```python
from build123d import *

# Parameters (mm, degrees)
F1_DEPTH = 20
F2_F1_R  = 2
F2_F2_R  = 2
F2_F3_R  = 2


with BuildPart() as f1:
    # F0 (on Top) → F1 (new body)
    with BuildSketch(Plane.XY):
        with BuildLine():
            ThreePointArc((0, 3.4753886408), (-6.702786735, 6.3139324677), (-9.1361551027, -0.5463444553))
            Line((-9.1361551027, -0.5463444553), (0, -18.3376532868))
            Line((0, -18.3376532868), (9.1361551027, -0.5463444553))
            ThreePointArc((9.1361551027, -0.5463444553), (6.702786735, 6.3139324677), (0, 3.4753886408))
        make_face()
        with BuildLine():
            ThreePointArc((0, 0), (-0.3116721052, 1.7376943204), (0, 3.4753886408))
            ThreePointArc((0, 3.4753886408), (0.3116721052, 1.7376943204), (0, 0))
        make_face(mode=Mode.SUBTRACT)
        with BuildLine():
            ThreePointArc((0, 0), (0.3116721052, 1.7376943204), (0, 3.4753886408))
            ThreePointArc((0, 3.4753886408), (-0.3116721052, 1.7376943204), (0, 0))
        make_face()
    extrude(amount=F1_DEPTH)

    # F2: fillet of radius 2 on 7 edges, made by hand

    # F2_f1
    f2_f1_edges = [f1.edges().sort_by_distance(p)[0] for p in [
        (0, 3.4753886408, 10),
    ]]
    fillet(f2_f1_edges, radius=F2_F1_R)

    # F2_f2
    f2_f2_edges = [f1.edges().sort_by_distance(p)[0] for p in [
        (0, -18.3376532868, 10),
    ]]
    fillet(f2_f2_edges, radius=F2_F2_R)

    # F2_f3
    f2_f3_edges = [f1.edges().sort_by_distance(p)[0] for p in [
        (7.7367258426, 5.7009341506, 0),
        (7.7367258426, 5.7009341506, 20),
        (5.4576429929, -7.7097019344, 0),
        (5.4576429929, -7.7097019344, 20),
        (0, -15.9594439033, 20),
        (0, -15.9594439033, 0),
        (1e-10, 4.9357306327, 20),
        (1e-10, 4.9357306327, 0),
    ]]
    fillet(f2_f3_edges, radius=F2_F3_R)


solid = f1.part
```
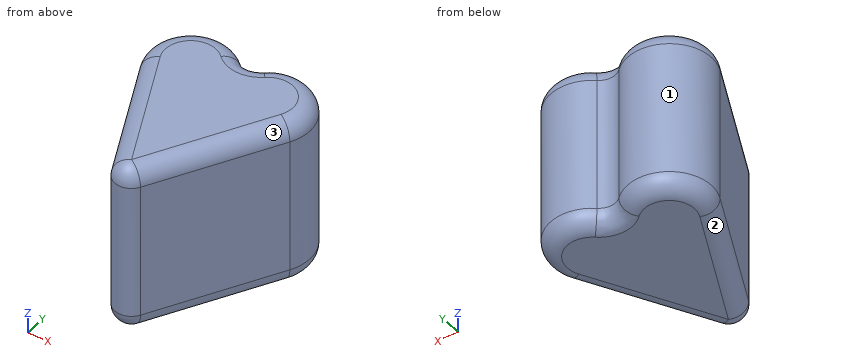
Geometry check sheet. Reference: the model listing, model coordinates, mm. Face numbers are marked on the shaded views. Give positions to 0.01 mm unless a question says otherwise; leave off trailing zeros. Use one line per item in the form item = value.
Item 1: Scan lines: line 1 (X direction, y = -7.5, z = 16.5); line 2 (Y direction, x = 4, z = 2.5); line 3 (Z direction, x = -6, y = 5). Record each from-to range of solid material in increasing order.
Results list:
line_1 = -5.57 to 5.57
line_2 = -10.55 to 6.69
line_3 = 0.07 to 19.93
Item 2: Mould release check, pull along X, two halves, no side actions. Record for the marked faces 1, 2 and 3: released by +X, released by -X, zero draft, split by the parting line, or undercut.
Results list:
face_1 = undercut
face_2 = released by -X
face_3 = released by +X
Item 3: Depth check by flat-ended pin: pin 1 Ø3 at (x, z) = (-4.5, 16.5) entering from -Y; pin 2 Ø1.5 at (x, z) = (7.5, 7) entering from +Y; pin 3 Ø10 at (x, y) = (-5.5, -5) entering from -Z; pin 4 Ø3 at (y, z) = (-8, 17) entering from -X. Enter the tip coordinate at first touch or a pass-through.
Results list:
pin_1 = -12.5
pin_2 = 6.29
pin_3 = 0
pin_4 = -6.08
